Geometry: see drawing. Coordinates: mm, zero at the bounding-box minimum. A direction names the side the tool comes from. Round coordinates to 2 decimals unless told otherwise and drop trailing zeros. Order: outer loops, then holes, each group sorted by start corner. A loop starts at its lowest first (then second) coordinate and runs counter-clockwise, first axis right, second up. Notation, with made-up numbers: (1.5, 29.5) -> (53.5, 29.5) arc R20 cw to (53.5, 36.5) -> close; hole circle Ø4 at (24, 45.25). An arc over 180 degrees is marked (long way). One line per item, written item: value. Start each with the question number.
1) Section B-B (z = 6.5). Return the cut outline in (x, y), and give its area (3 significant figures).
2) Pin query (flat end, axial travel): P1, Ø3, axis at y = 16.5, z = 6.5, coming from the +X side; P2, Ø4, axis at y = 12.5, z = 4.5, coming from the -X side. Return the tip coordinate at first contact, or that it passes through.
3) Reachability of the marked faces 1 and 2 from +Z, -Z, +X, -X, +Y, -Y: full face, straight path, thin tool, end or side. Return the list, or none.
4) Mould query, pull axis Z, two halves, no side actions, for the marked faces 3, 4 and 5. Classes: pulls with the +Z half, pulls with the -Z half, needs draft (parallel to the pull), parting line crosses it, or undercut.
5) Section D-D (z = 1). Return the cut outline in (x, y), and give its area (3 significant figures).
6) Section A-A (y = 7). Return the cut outline in (x, z), and give its area (3 significant figures).
7) Ray query, L1, parallel to Y at x = 5, z = 2.65; L2, parallel to Y at x = 5, z = 8.5. Return the intervals inside material, ascending.
8) Section C-C (x = 3.25). Return the cut outline in (y, z).
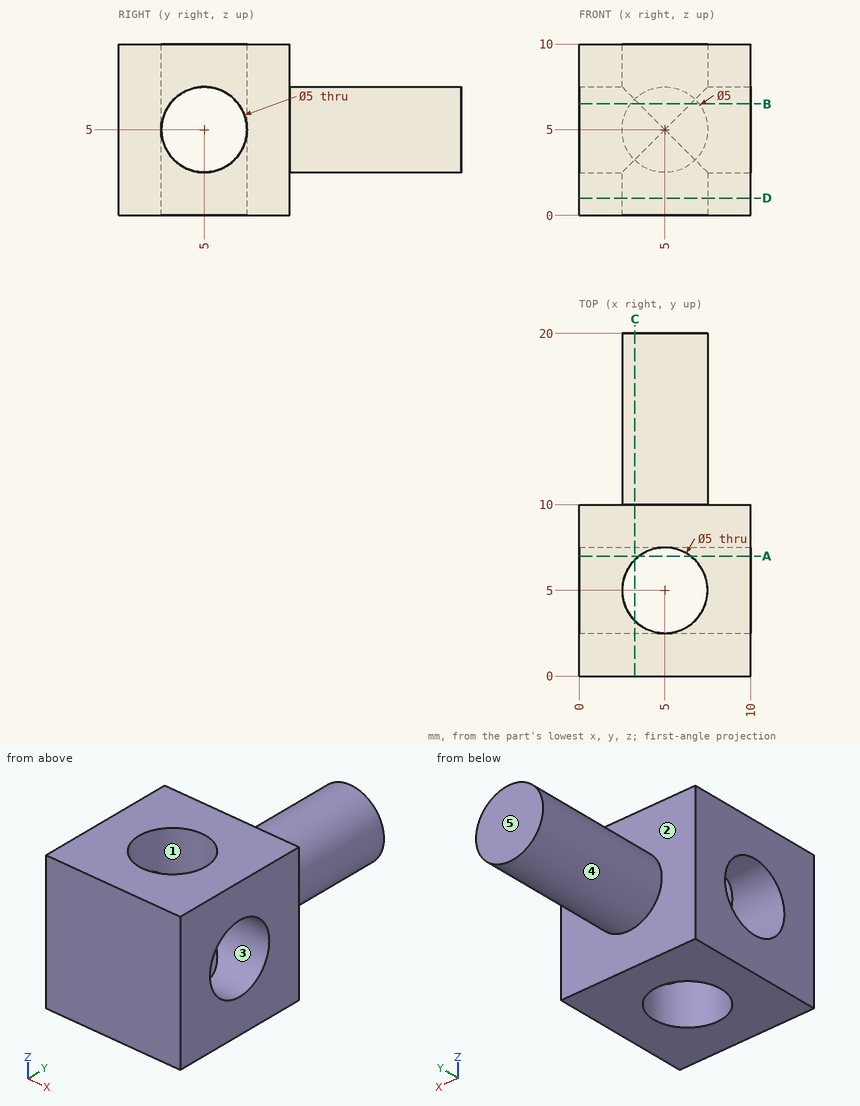
Findings:
1. outline: (0, 0) -> (10, 0) -> (10, 3) -> (6.5, 3) arc R2.5 cw to (3.5, 3) -> (0, 3) -> close; (0, 7) -> (3.5, 7) arc R2.5 cw to (6.5, 7) -> (10, 7) -> (10, 10) -> (7, 10) -> (7, 20) -> (3, 20) -> (3, 10) -> (0, 10) -> close
1. area: 98.0 mm2
2. P1: x = 7.5
2. P2: x = 2.5
3. face 1: +Z, -Z
3. face 2: +Y
4. face 3: undercut
4. face 4: parting line crosses it
4. face 5: needs draft
5. outline: (0, 0) -> (10, 0) -> (10, 10) -> (0, 10) -> close; hole circle Ø5 at (5, 5)
5. area: 80.4 mm2
6. outline: (0, 0) -> (3.5, 0) -> (3.5, 3.5) -> (0, 3.5) -> close; (0, 6.5) -> (3.5, 6.5) -> (3.5, 10) -> (0, 10) -> close; (6.5, 0) -> (10, 0) -> (10, 3.5) -> (6.5, 3.5) -> close; (6.5, 6.5) -> (10, 6.5) -> (10, 10) -> (6.5, 10) -> close
6. area: 49.0 mm2
7. L1: 0 to 2.5, 7.5 to 20
7. L2: 0 to 2.5, 7.5 to 10
8. outline: (0, 0) -> (3.21, 0) -> (3.21, 3.25) arc R2.5 cw to (3.21, 6.75) -> (3.21, 10) -> (0, 10) -> close; (6.79, 0) -> (10, 0) -> (10, 3.21) -> (20, 3.21) -> (20, 6.79) -> (10, 6.79) -> (10, 10) -> (6.79, 10) -> (6.79, 6.75) arc R2.5 cw to (6.79, 3.25) -> close
